Geometry: final body of the model. Coordinates: model frame, mm. A direction names the side the tool comes from. Round coordinates to 2 decimals unless told otherwise and drop trailing zeros. Write each loop counter-clockwise with the first axis right and the second up, starting at its lowest first coordinate (ties: lowest second). Pieces come first, ordered by that corner, then holes. Notation, with made-up numbers: M -14.5,5 L 28.5,5 A13 ccw 28.5,19 Z; hole C 13.25,63 d11. An arc over 180 degrees is marked long. Put each result on its own line as item: value. Start each with the question number.
```python
from build123d import *

# Parameters (mm, degrees)
F0_W          = 160
F0_H          = 60
F0_R          = 10
F1_DEPTH      = 15
F3_DEPTH      = 30
F3_DEPTH_BACK = 30
F4_T1_DEPTH   = 407.2453152316
F5_R          = 34.99999


# Not quite as in the source:
# - a fillet or chamfer that OpenCascade refuses, or shapes differently, is made with other operations: its cross-section is extruded or revolved along the edge and cut away or added
# - a fillet or chamfer is up to 0.001 mm smaller than in the source, because OpenCascade refuses the exact size


with BuildPart() as f1:
    # F0 (on Top) → F1 (new body)
    with BuildSketch(Plane.XY):
        Rectangle(F0_W, F0_H)
        with Locations((-57.5, 0)):
            Circle(F0_R, mode=Mode.SUBTRACT)
        with Locations((57.5, 0)):
            Circle(F0_R, mode=Mode.SUBTRACT)
    extrude(amount=F1_DEPTH)

    # F2 (on Front) → F3 (join, two sides)
    with BuildSketch(Plane.XZ) as f3_sk:
        with BuildLine():
            Line((35.0165497145, 49.646243304), (17.5165497145, 49.646243304))
            ThreePointArc((17.5165497145, 49.646243304), (0.0165497145, 32.146243304), (-17.4834502855, 49.646243304))
            Line((-17.4834502855, 49.646243304), (-34.9834502855, 49.646243304))
            Line((-34.9834502855, 49.646243304), (-34.9834502855, 14.646243304))
            Line((-34.9834502855, 14.646243304), (35.0165497145, 14.646243304))
            Line((35.0165497145, 14.646243304), (35.0165497145, 49.646243304))
        make_face()
        with BuildLine():
            ThreePointArc((-17.4834502855, 49.646243304), (0.0165497145, 67.146243304), (17.5165497145, 49.646243304))
            Line((17.5165497145, 49.646243304), (35.0165497145, 49.646243304))
            Line((35.0165497145, 49.646243304), (35.0165497145, 54.9693842517))
            Line((35.0165497145, 54.9693842517), (35.0165497145, 84.646243304))
            Line((35.0165497145, 84.646243304), (-34.9834502855, 84.646243304))
            Line((-34.9834502855, 84.646243304), (-34.9834502855, 49.646243304))
            Line((-34.9834502855, 49.646243304), (-17.4834502855, 49.646243304))
        make_face()
    extrude(amount=F3_DEPTH)
    extrude(f3_sk.sketch, amount=-F3_DEPTH_BACK)

    # F4: chamfer of 65 x 23.6580652273 on 1 edges, made by hand

    # F4_s2 → F4_t1 (cut)
    with BuildSketch(Plane.YZ.offset(-203.6061079013)):
        Polygon((-30, 19.646243304), (-6.3419347727, 84.646243304), (-30, 84.646243304), align=None)
    extrude(amount=F4_T1_DEPTH, mode=Mode.SUBTRACT)

    # F5 (radius 35 in the source; OpenCascade refuses exactly that, so slightly less here)
    f5_edges = [f1.edges().sort_by_distance(p)[0] for p in [
        (35.01655, 11.829033, 84.646243),
        (-34.98345, 11.829033, 84.646243),
    ]]
    fillet(f5_edges, radius=F5_R)


solid = f1.part
```
1) Section B-B, the plane x = 57.5. Output: boundary loops of the cut face in (y, z).
2) First-contact query: pin 1 (4 mm diameter, centred on y = 6, z = 45.5, fed in from -X); pin 2 (6 mm diameter, centred on y = 4.5, z = 59.5, fed in from +X); pin 3 (1.5 mm diameter, centred on x = 38, y = -4, fed in from +Z); pin 4 (2 mm diameter, centred on y = -22.5, z = 48, fed in from -X). Flat tips, straight axial feed; report the tip coordinate or a pass-through.
3) Access query for faces 1 (the face through (47, 0, 15)), 2 (the face through (80, 0, 7)), 3 (the face through (-68, 0, 15)). Directions: +Z, -Z, +X, -X, +Y, -Y. A direction counts if a zero-diameter tool reaches every point of the face in a straight line with its end or side. Return the directions, or none.
4) Section D-D, the plane z = 38.5. Output: boundary loops of the cut face in (x, y), and give its area (3 significant figures).
5) Section A-A, the plane y = 0. Give the number of separate pieces and of enclosed holes in the cut face, and give its area (3 significant figures).
6) Draft query along X for faces 4 (the face through (-34.983, 0, 33)), 5 (the face through (47.51, 0.44, 7.4)), 6 (the face through (-1, 0, 0)). Return one class per face: +X half, -X half, draft (parallel to the pull), parting line (faces both ways), or undercut.
7) Ray query, probe 1 along X at (y, z) = (5, 11); probe 2 along Z at (x, y) = (-64.5, 11); probe 3 along X at (y, z) = (12, 31). Return the intervals inside material, ascending.
Solved:
1. outline: M -30,0 L -10,0 L -10,15 L -30,15 Z; M 10,0 L 30,0 L 30,15 L 10,15 Z
2. pin 1: stops at x = -34.98
2. pin 2: stops at x = 34.34
2. pin 3: stops at z = 15
2. pin 4: passes through
3. face 1: +Z, +X, +Y, -Y
3. face 2: +Z, -Z, +X, +Y, -Y
3. face 3: +Z, -X, +Y, -Y
4. outline: M -34.98,-23.14 L -13.47,-23.14 L -13.47,30 L -34.98,30 Z; M 13.51,-23.14 L 35.02,-23.14 L 35.02,30 L 13.51,30 Z
4. area: 2,290 mm2
5. separate pieces: 3
5. enclosed holes: 1
5. area: 5,190 mm2
6. face 4: -X half
6. face 5: undercut
6. face 6: draft
7. probe 1: x = -80 to -66.16, -48.84 to 48.84, 66.16 to 80
7. probe 2: z = 0 to 15
7. probe 3: x = -34.98 to 35.02
